```python
from build123d import *

# Parameters (mm, degrees)
F1_DEPTH       = 12.7
F3_DEPTH       = 6.35
F5_D           = 7.1374
F5_CSINK_D     = 13.4874
F5_CSINK_ANGLE = 82


with BuildPart() as f1:
    # F0 (on Top) → F1 (new body)
    with BuildSketch(Plane.XY):
        with BuildLine():
            Line((-177.8, 0), (-152.4, 0))
            ThreePointArc((-152.4, 0), (0, 152.4), (152.4, 0))
            Line((152.4, 0), (177.8, 0))
            ThreePointArc((177.8, 0), (0, 177.8), (-177.8, 0))
        make_face()
    extrude(amount=F1_DEPTH)

    # F2 (on face) → F3 (join)
    with BuildSketch(Plane(origin=(0, 0, 0), x_dir=(1, 0, 0), z_dir=(0, 0, -1))):
        with BuildLine():
            Line((-164.6108137396, -12.7), (-151.9108137396, -12.7))
            ThreePointArc((-151.9108137396, -12.7), (-151.9202246619, -12.2111760422), (-151.9484434816, -11.7230765386))
            ThreePointArc((-151.9484434816, -11.7230765386), (-155.9828628767, -3.3807476744), (-164.6108137281, 0))
            ThreePointArc((-164.6108137281, 0), (-173.5910698566, -3.7197438749), (-177.3108137396, -12.7))
            Line((-177.3108137396, -12.7), (-164.6108137396, -12.7))
        make_face()
        with BuildLine():
            ThreePointArc((151.9484434411, -11.7230770637), (151.9202246518, -12.2111763053), (151.9108137396, -12.7))
            Line((151.9108137396, -12.7), (177.3108137396, -12.7))
            ThreePointArc((177.3108137396, -12.7), (173.5910698566, -3.7197438749), (164.6108137281, 0))
            ThreePointArc((164.6108137281, 0), (155.9828626834, -3.3807478534), (151.9484434411, -11.7230770637))
        make_face()
    extrude(amount=F3_DEPTH)

    # F5 (through all)
    with Locations(Plane(origin=(0, 0, 0), x_dir=(1, 0, 0), z_dir=(0, 0, -1))):
        with Locations((-142.9807941648, -82.55), (-82.55, -142.9807941648), (0, -165.1), (82.55, -142.9807941648), (142.9807941648, -82.55)):
            CounterSinkHole(F5_D / 2, F5_CSINK_D / 2, counter_sink_angle=F5_CSINK_ANGLE)


solid = f1.part
```
Part model, mm, in its own coordinate system. A direction names the side the tool comes from. Round coordinates to 2 decimals unless told otherwise and drop trailing zeros. Loops run counter-clockwise (first coordinate to the right, second up) from the corner with the lowest first, then second, coordinate; pieces in that order, holes last. Notation, with made-up numbers: (42.25, 7) -> (70.25, 7) arc R19 cw to (70.25, 14) -> close; hole circle Ø5 at (47, 64). An arc over 180 degrees is marked (long way). Use CSV: the item, a comma, the result in double quotes. Start each with the question number.
1) Cut at B-B, the plane y = 27.5. Write the cut outline in (x, z), plus the area to 3 significant figures.
2) Wall check: L1, parallel to X at y = 82.55, z = 6.5; L2, parallel to Y at x = 0, z = 7.75; L3, parallel to Z at x = 152.5, y = 42. Give the ranges that are in metal, low to high. Write a range as [from, to].
3) Cut at C-C, the plane y = 57.5. Write the cut outline in (x, z), plus the area to 3 significant figures.
4) Pull direction Y, two halves, no side cores. Call faces 4 (the flat face through (-165, 0, 6)), 5 (the cylindrical face through (3.91, 177.757, 6.261)), 6 (the flat face through (-1, 155, 0)), 7 (the cylindrical face through (-79.92, 140.57, 8.24)): +Y half, -Y half, draft (parallel to the pull), parting line (faces both ways), or undercut.
5) Cut at A-A, the plane x = 0. Write the cut outline in (y, z), plus the area to 3 significant figures.
6) Cut at D-D, the plane x = -82.55. Write the cut outline in (y, z), plus the area to 3 significant figures.
7) Drop flat-ended pins along their axis: P1, Ø1.5, axis at y = 88, z = -2, coming from the -X side; P2, Ø10, axis at x = 106, z = -1, coming from the +Y side; P3, Ø1.5, axis at y = 105, z = 9, coming from the -X side; P4, Ø8, axis at x = -123.5, z = 10.5, coming from the -Y side. Give the stop position or say it passes through.
8) Which spindle directions (+Z, -Z, +X, -X, +Y, -Y) get a long thin tool onto all of the face, cutting with end or side? Do faces 1 (the flat face through (164, 12.7, -3)), 2 (the flat face through (155, 3, 0)), 3 (the conical face through (145.935, 84.815, 3.475)). Say none if no direction does.
Determined:
1,outline,"(-175.66, 0) -> (-149.9, 0) -> (-149.9, 12.7) -> (-175.66, 12.7) -> close; (149.9, 0) -> (175.66, 0) -> (175.66, 12.7) -> (149.9, 12.7) -> close"
1,area,"654 mm2"
2,L1,"x = [-157.47, -146.55], [-139.41, -128.11], [128.11, 139.41], [146.55, 157.47]"
2,L2,"y = [152.4, 161.53], [168.67, 177.8]"
2,L3,"z = [0, 12.7]"
3,outline,"(-168.25, 0) -> (-141.14, 0) -> (-141.14, 12.7) -> (-168.25, 12.7) -> close; (141.14, 0) -> (168.25, 0) -> (168.25, 12.7) -> (141.14, 12.7) -> close"
3,area,"689 mm2"
4,face 4,"-Y half"
4,face 5,"+Y half"
4,face 6,"draft"
4,face 7,"undercut"
5,outline,"(152.4, 0) -> (158.36, 0) -> (161.53, 3.65) -> (161.53, 12.7) -> (152.4, 12.7) -> close; (168.67, 3.65) -> (171.84, 0) -> (177.8, 0) -> (177.8, 12.7) -> (168.67, 12.7) -> close"
5,area,"220 mm2"
6,outline,"(128.11, 0) -> (136.24, 0) -> (139.41, 3.65) -> (139.41, 12.7) -> (128.11, 12.7) -> close; (146.55, 3.65) -> (149.72, 0) -> (157.47, 0) -> (157.47, 12.7) -> (146.55, 12.7) -> close"
6,area,"271 mm2"
7,P1,"passes through"
7,P2,"stops at y = 146.26"
7,P3,"stops at x = -144.03"
7,P4,"stops at y = 83.48"
8,face 1,"-Z, +X, -X, +Y"
8,face 2,"-Z, -Y"
8,face 3,"-Z"
